Autodesk Inventor part; units mm, degrees
ref_plane "YZ Plane" through (0, 0, 0) normal (1, 0, 0) x (0, 1, 0)
ref_plane "XZ Plane" through (0, 0, 0) normal (0, 1, 0) x (-1, 0, 0)
ref_plane "XY Plane" through (0, 0, 0) normal (0, 0, 1) x (1, 0, 0)
sketch "Sketch1" plane through (0, 0, 0) normal (0, 1, 0) x (-1, 0, 0)
  circle A0 centre (-55, 20) radius 2.75
  circle A1 centre (-55, -20) radius 2.75
  circle A2 centre (-55, 20) radius 8
  circle A3 centre (-55, -20) radius 8
  circle A4 centre (-25.5769, 0) radius 21
  line L0 (-55.1769, 10.2) -> (-14.5769, 10.2)
  line L1 (-14.5769, 10.2) -> (-14.5769, -10.2)
  line L2 (-14.5769, -10.2) -> (-55.1769, -10.2)
  line L3 (-55.1769, -10.2) -> (-55.1769, 10.2)
  line L4 (-14.5769, 10.2) -> (-7.7769, 10.2)
  line L5 (-7.7769, 10.2) -> (-7.7769, -10.2)
  line L6 (-7.7769, -10.2) -> (-14.5769, -10.2)
  line L7 (-14.5769, -10.2) -> (-14.5769, 10.2)
  line L8 (-55.1769, 10.2) -> (-61.9769, 10.2)
  line L9 (-61.9769, 10.2) -> (-61.9769, -10.2)
  line L10 (-61.9769, -10.2) -> (-55.1769, -10.2)
  line L11 (-55.1769, -10.2) -> (-55.1769, 10.2)
  circle A5 centre (-9.5857, -4.75) radius 2.5
  circle A6 centre (-9.5857, 4.75) radius 2.5
  line L12 (-9.5857, 4.75) -> (-9.5857, -4.75)
  line L13 (-9.5857, -10.2) -> (-9.5857, -4.75)
  line L14 (-9.5857, 4.75) -> (-9.5857, 10.2)
  line L15 (-25.5769, 10.2) -> (-25.5769, 21)
  line L16 (-25.5769, -10.2) -> (-25.5769, -21)
  line L17 (-25.5769, 0) -> (-55.1769, 0)
  line L18 (13.335, 0) -> (-80.01, 0)
  line L19 (0, -46.4332) -> (0, 45.2366)
  line L20 (-4.5769, 0) -> (-7.7769, 0)
  circle A7 centre (-25.5769, 0) radius 18.1
  circle A8 centre (-55, 20) radius 6
  circle A9 centre (-55, -20) radius 5.6406
  circle A10 centre (-58.7982, -4.75) radius 2.5
  circle A11 centre (-58.7982, 4.75) radius 2.5
  line L21 (-2.7857, 32.1409) -> (-66.675, 32.1409)
  line L22 (-66.675, 32.1409) -> (-66.675, -33.3375)
  line L23 (-66.675, -33.3375) -> (-2.7857, -33.3375)
  line L24 (-2.7857, -33.3375) -> (-2.7857, 32.1409)
  line L25 (-6.1769, 12) -> (-63.8933, 12)
  line L26 (-63.8933, 12) -> (-63.8933, -12)
  line L27 (-63.8933, -12) -> (-6.1769, -12)
  line L28 (-6.1769, -12) -> (-6.1769, 12)
  circle A12 centre (-55, -20) radius 1.75
  circle A13 centre (-55, 20) radius 1.75
  line L29 (-49, 32.1409) -> (-49, 20)
  point P0 (0, 0)
  point P1 (-8.5769, -5.0781)
  dimension "d23" = 12
  dimension "d56" = -0.2
  dimension "d0" = 5.5
  dimension "d1" = 5.5
  dimension "d2" = 16
  dimension "d3" = 16
  dimension "d5" = 42
  dimension "d6" = 40.6
  dimension "d7" = 20.4
  dimension "d8" = 6.8
  dimension "d9" = 6.8
  dimension "d10" = 5
  dimension "d11" = 5
  dimension "d16" = 9.5
  dimension "d17" = 29.6
  dimension "d20" = -55
  dimension "d21" = -55
  dimension "d22" = 36.2
  dimension "d24" = 5
  dimension "d25" = 5
  dimension "d26" = 9.5
  dimension "d27" = 20
  dimension "d28" = 20
  dimension "d31" = 1
extrude "Extrusion1" add sketch "Sketch1" along normal blind 10 contours A0 | A1 | A2 | A2 L29 L21 L24 L18 A4 L28 L25 | A2 L25 L26 L18 L22 L21 L29 | L25 A4 L0 L8 L9 L18 L26 | L25 A7 L0 A4 | A4 L15 A7 L25 | A4 L25 A7 L15 | L25 L15 L0 A7 | A7 L15 L25 | A3 | L26 L27 A4 L28 L18 L24 L23 L22 | L18 L9 L10 L2 A4 L27 L26 | L25 L28 A4 | A4 L28 L18 A7 A6 L5 L4 L25 | A7 L25 L15 | L3 L18 L9 L8 | L25 A7 L4 L0 L15 | L18 L3 L10 L9 | L18 L28 A4 | A4 L28 L18 | L2 A7 L27 A4 | L28 L27 A4 | A4 L27 A7 L6 L5 A5 L18 L28 | A7 L14 A6 L12 L18 L1 L4 | L4 L14 A7 | L27 A7 L16 A4 | L2 L16 L27 A7 | A4 L16 A7 L27 | A7 A5 L5 L18 | L18 L5 A6 A7 | L4 L5 A6 A7 L14 | A7 A6 L14 | L27 L16 A7 | L2 L6 A7 L27 L16 | L18 L12 A5 L13 A7 L6 L1 | A7 L16 L27 | L18 L12 A6 L5 | L5 A5 L12 L18 | A7 L13 L6 | L13 A7 A5 L5 L6 | L13 A5 A7 | A8 | A9 | A12 | A13
extrude "Extrusion2" add sketch "Sketch1" along normal blind 30 from surface at 10 contours A12 | A13
move faces "Move5" translate (0, 0, 0.2) faces at (41.6436, 6.6667, 10.2)
move faces "Move6" translate (0, 0, -0.2) faces at (28.1103, 6.6667, -10.2)
move faces "Move7" translate (0.2, 0, 0) faces at (55.1769, 3.3333, -3.4667)
move faces "Move8" translate (-0.2, 0, 0) faces at (14.5769, 3.3333, 3.4667)
sketch "Sketch2" plane through (2.7857, 0, -33.3375) normal (-1, 0, 0) x (0, 0, 1)
  line L0 (0, 0) -> (0, 10)
  line L1 (55.5625, 0) -> (55.5625, -40.2602)
  line L2 (0, 0) -> (65.4784, 0)
  line L3 (23.8125, 0) -> (23.8125, -55)
  line L4 (0, 0) -> (10, 0)
  line L5 (10, 0) -> (10, -50)
  line L6 (10, -50) -> (0, -50)
  line L7 (0, -50) -> (0, 0)
  line L8 (10, -50) -> (45.3991, -70.4377)
  line L9 (45.3991, -70.4377) -> (45.3991, -76.2112)
  line L10 (45.3991, -76.2112) -> (0, -50)
  line L11 (26.0875, 10) -> (26.0875, 0)
  line L12 (65.4784, 0) -> (65.4784, 10)
  line L13 (0, 10) -> (65.4784, 10)
  line L14 (0, 0) -> (65.4784, 0)
  line L15 (65.4784, 0) -> (65.4784, 10)
  line L16 (0, 10) -> (65.4784, 10)
  line L17 (0, 0) -> (0, 10)
  line L18 (35.5875, 0) -> (40.5875, 0)
  line L19 (26.0875, 10) -> (31.0875, 10)
  line L20 (26.0875, 0) -> (31.0875, 0)
  line L21 (26.0875, 0) -> (31.0875, 0)
  line L22 (43.7375, 0) -> (22.9375, 0)
  line L23 (22.9375, 0) -> (22.9375, 10)
  line L24 (43.7375, 10) -> (22.9375, 10)
  line L25 (43.7375, 0) -> (43.7375, 10)
  line L26 (43.7375, 0) -> (22.9375, 0)
  line L27 (22.9375, 0) -> (22.9375, 10)
  line L28 (43.7375, 10) -> (22.9375, 10)
  line L29 (43.7375, 0) -> (43.7375, 10)
  line L30 (65.4784, 0) -> (65.4784, 10)
  line L31 (65.4784, 0) -> (65.4784, 10)
  line L32 (65.4784, 0) -> (65.4784, 10)
  line L33 (51.5875, 10) -> (55.0875, 10)
  line L34 (11.5875, 10) -> (15.0875, 10)
  line L35 (65.4784, 10) -> (0, 10)
  line L36 (0, 10) -> (65.4784, 10)
  line L37 (35.5875, 10) -> (40.5875, 10)
  line L38 (43.7375, 10) -> (22.9375, 10)
  line L39 (22.9375, 10) -> (43.7375, 10)
  line L40 (35.5875, 10) -> (40.5875, 10)
  line L41 (26.0875, 10) -> (31.0875, 10)
  line L42 (26.0875, 10) -> (31.0875, 10)
  line L43 (0, 0) -> (65.4784, 0)
  line L44 (65.4784, 0) -> (0, 0)
  line L45 (35.5875, 0) -> (40.5875, 0)
  line L46 (43.7375, 0) -> (22.9375, 0)
  line L47 (22.9375, 0) -> (43.7375, 0)
  line L48 (35.5875, 0) -> (40.5875, 0)
  line L49 (26.0875, 0) -> (31.0875, 0)
  line L50 (26.0875, 0) -> (31.0875, 0)
  line L51 (65.4784, 10) -> (0, 10)
  line L52 (65.4784, 0) -> (0, 0)
  line L53 (0, 0) -> (0, 10)
  line L54 (65.4784, 10) -> (0, 10)
  line L55 (65.4784, 0) -> (65.4784, 10)
  line L56 (65.4784, 0) -> (0, 0)
  line L57 (51.5875, 10) -> (55.0875, 10)
  line L58 (43.7375, 0) -> (43.7375, 10)
  line L59 (43.7375, 0) -> (43.7375, 10)
  line L60 (0, 0) -> (0, 10)
  line L61 (0, 0) -> (0, 10)
  line L62 (0, 0) -> (0, 10)
  line L63 (22.9375, 0) -> (22.9375, 10)
  line L64 (22.9375, 0) -> (22.9375, 10)
  line L65 (26.0875, 10) -> (31.0875, 10)
  line L66 (26.0875, 0) -> (31.0875, 0)
  line L67 (43.7375, 0) -> (43.7375, 10)
  line L68 (22.9375, 0) -> (22.9375, 10)
  line L69 (22.9375, 0) -> (43.7375, 0)
  line L70 (22.9375, 0) -> (43.7375, 0)
  line L71 (43.7375, 0) -> (43.7375, 10)
  line L72 (22.9375, 10) -> (43.7375, 10)
  line L73 (22.9375, 0) -> (22.9375, 10)
  line L74 (35.5875, 10) -> (40.5875, 10)
  line L75 (35.5875, 10) -> (40.5875, 10)
  line L76 (35.5875, 0) -> (40.5875, 0)
  line L77 (22.9375, 10) -> (43.7375, 10)
  line L78 (26.0875, 10) -> (31.0875, 10)
  line L79 (51.5875, 10) -> (55.0875, 10)
  line L80 (51.5875, 40) -> (55.0875, 40)
  line L81 (51.5875, 40) -> (55.0875, 40)
  line L82 (51.5875, 40) -> (55.0875, 40)
  line L83 (35.5875, 10) -> (40.5875, 10)
  line L84 (35.5875, 0) -> (40.5875, 0)
  line L85 (35.5875, 10) -> (40.5875, 10)
  line L86 (26.0875, 10) -> (31.0875, 10)
  line L87 (35.5875, 0) -> (40.5875, 0)
  line L88 (26.0875, 0) -> (31.0875, 0)
  line L89 (11.5875, 10) -> (15.0875, 10)
  line L90 (11.5875, 40) -> (15.0875, 40)
  line L91 (11.5875, 40) -> (15.0875, 40)
  line L92 (11.5875, 10) -> (15.0875, 10)
  line L93 (11.5875, 40) -> (15.0875, 40)
  line L94 (-13.0957, 0) -> (78.5741, 0)
  point P0 (33.3375, 0)
  point P1 (10, 0)
  dimension "d63" = 55
  dimension "d64" = 10
  dimension "d65" = 120
  dimension "d66" = 120
  dimension "d102" = 50
extrude "Extrusion3" add sketch "Sketch2" against normal blind 65.5625 contours L2 L5 L6 L7 | L6 L8 L9 L10
move faces "Move9" translate (-1.588, 0, 0) faces at (68.3482, -16.6667, -30.0042) (27.9459, 0, 24.8939)
sketch "Sketch3" plane through (2.7857, -50, -33.3375) normal (0, -0.8660254, -0.5) x (1, 0, 0)
  circle A0 centre (57, 36.7033) radius 1.75
  circle A1 centre (47, 36.7033) radius 1.75
  circle A2 centre (37, 36.7033) radius 1.75
  line L0 (57, 36.7033) -> (47, 36.7033)
  line L1 (37, 36.7033) -> (47, 36.7033)
  circle A3 centre (57, 26.7033) radius 1.75
  circle A4 centre (47, 26.7033) radius 1.75
  circle A5 centre (37, 26.7033) radius 1.75
  line L2 (57, 26.7033) -> (47, 26.7033)
  line L3 (37, 26.7033) -> (47, 26.7033)
  circle A6 centre (57, 16.7033) radius 1.75
  circle A7 centre (47, 16.7033) radius 1.75
  circle A8 centre (37, 16.7033) radius 1.75
  line L4 (57, 16.7033) -> (47, 16.7033)
  line L5 (37, 16.7033) -> (47, 16.7033)
  circle A9 centre (27, 16.7033) radius 1.75
  circle A10 centre (17, 16.7033) radius 1.75
  circle A11 centre (7, 16.7033) radius 1.75
  line L6 (27, 16.7033) -> (17, 16.7033)
  line L7 (7, 16.7033) -> (17, 16.7033)
  circle A12 centre (27, 36.7033) radius 1.75
  circle A13 centre (17, 36.7033) radius 1.75
  circle A14 centre (7, 36.7033) radius 1.75
  line L8 (27, 36.7033) -> (17, 36.7033)
  line L9 (7, 36.7033) -> (17, 36.7033)
  circle A15 centre (27, 26.7033) radius 1.75
  circle A16 centre (17, 26.7033) radius 1.75
  circle A17 centre (7, 26.7033) radius 1.75
  line L10 (27, 26.7033) -> (17, 26.7033)
  line L11 (7, 26.7033) -> (17, 26.7033)
  line L12 (58.75, 36.7033) -> (64.329, 36.7033)
  line L13 (0, 49.5356) -> (0, 8.6603)
  line L14 (0, 36.7033) -> (7, 36.7033)
  point P0 (-2.7857, 3.8711)
  dimension "d72" = 3.5
  dimension "d73" = 10
  dimension "d74" = 3.5
  dimension "d75" = 10
  dimension "d76" = 0
  dimension "d77" = 10
  dimension "d78" = 3.5
  dimension "d79" = 10
  dimension "d84" = 3.5
  dimension "d85" = 10
  dimension "d90" = 3.5
  dimension "d91" = 10
  dimension "d92" = 3.5
  dimension "d93" = 10
  dimension "d94" = 0
  dimension "d95" = 10
  dimension "d96" = 10
  dimension "d97" = 10
  dimension "d98" = 10
  dimension "d101" = 7
extrude "Extrusion4" cut sketch "Sketch3" against normal blind 30
Design review of the part built by this model. Coordinates are the model's own, in mm. A direction names the side the tool comes from. Round coordinates to 2 decimals unless told otherwise and drop trailing zeros. Order: outer loops, then holes, each group sorted by start corner. A loop starts at its lowest first (then second) coordinate and runs counter-clockwise, first axis right, second up. Notation, with made-up numbers: M 74.5,11 L 104.5,11 A35 ccw 104.5,46 Z; hole C 45,18.25 d7. An arc over 180 degrees is marked long. Answer as CSV lines item,"result". Start each with the question number.
1) Tool access review of faces 1 (the face through (53.331, 24.79, 19.474)), 2 (the face through (34.325, -60.076, -5.886)), 3 (the face through (11.455, -61.48, -8.524)): name each direction out of +Z, -Z, +X, -X, +Y, -Y from which nothing blocks a thin tool from reaching the whole face with its end or side.
2) Add section A-A (y = 1.5). Give the number of separate pieces and of enclosed holes in the cut face, then the cut area to 3 significant figures.
3) Add section C-C (z = 20). Give the boundary of the cut face in (x, y) (3 decimals), then the cut area to 3 significant figures.
4) Add section B-B (z = -4.75). Give the boundary of the cut face in (x, y) (1 decimal), then the cut area to 3 significant figures.
5) The part is to be moulded in two halves that separate along Y. For faces 4 (the face through (66.675, 5, 0)), 5 (the face through (34.3, -63.3, -10.3)), 6 (the face through (61.4, -55.88, -18.22)), say which applies: +Y half, -Y half, draft (parallel to the pull), parting line (faces both ways), or undercut.
6) Add section D-D (y = 31). Give the boundary of the cut face in (x, z), then the cut area to 3 significant figures.
7) Wall thickness on line 1 along X through (y, z) = (4.25, 4.75) (3 decimals); line 2 along X through (y, z) = (5, -4) (3 decimals); line 3 along Z through (x, y) = (59, -1.5): over which ranges is each line inside the solid? List them lowest first. Write a range as [from, to].
8) For pin 1 Ø12 at (x, y) = (58.5, -13) entering from +Z; pin 2 Ø4 at (x, z) = (58.8, 4.75) entering from -Y; pin 3 Ø16.5 at (x, z) = (44.5, -7) entering from -Y, all flat-tipped, find the tip position at first contact; note any pin that passes through.
Resolved:
1,face 1,"+Y"
1,face 2,"+Z, +X, -X"
1,face 3,"none"
2,separate pieces,"1"
2,enclosed holes,"5"
2,area,"3,250 mm^2"
3,outline,"M 2.786,0 L 66.675,0 L 66.675,10 L 56.75,10 L 56.75,40 L 53.25,40 L 53.25,10 L 2.786,10 Z"
3,area,"744 mm^2"
4,outline,"M 2.8,-66.5 L 66.8,-66.5 L 66.8,-60.7 L 2.8,-60.7 Z; M 2.8,0 L 7.1,0 L 7.1,10 L 2.8,10 Z; M 12.1,0 L 14.4,0 L 14.4,10 L 12.1,10 Z; M 55.4,0 L 56.3,0 L 56.3,10 L 55.4,10 Z; M 61.3,0 L 66.7,0 L 66.7,10 L 61.3,10 Z"
4,area,"498 mm^2"
5,face 4,"draft"
5,face 5,"-Y half"
5,face 6,"undercut"
6,outline,"C 55,-20 d3.5; C 55,20 d3.5"
6,area,"19.2 mm^2"
7,line 1,"[2.786, 7.086], [12.086, 14.377], [55.377, 56.298], [61.298, 66.675]"
7,line 2,"[2.786, 7.201], [11.971, 14.377], [55.377, 56.413], [61.183, 66.675]"
7,line 3,"[-33.34, -23.34]"
8,pin 1,"z = -23.34"
8,pin 2,"y = -73.14"
8,pin 3,"y = -69.97"
